```python
from build123d import *

# Parameters (mm, degrees)
PAD_DEPTH    = 6
PAD001_DEPTH = 5
SKETCH002_R  = 25
PAD002_DEPTH = 3
SKETCH003_R  = 20
PAD003_DEPTH = 12
FILLET_R     = 2


with BuildPart() as part:
    # Sketch → Pad (new body)
    with BuildSketch(Plane.XY):
        with BuildLine():
            Line((-1.45, 1.377498), (-1.45, -1.377498))
            ThreePointArc((-1.45, -1.377498), (0, -1.942662), (1.45, -1.377498))
            Line((1.45, 1.377498), (1.45, -1.377498))
            ThreePointArc((1.45, 1.377498), (0, 1.942662), (-1.45, 1.377498))
        make_face()
    extrude(amount=-PAD_DEPTH)

    # Sketch001 → Pad001 (join)
    with BuildSketch(Plane.XY):
        with BuildLine():
            Line((-8.25, 0), (0, 8.25))
            ThreePointArc((-8.25, 0), (5.833631, -5.833631), (0, 8.25))
        make_face()
    extrude(amount=PAD001_DEPTH)

    # Sketch002 → Pad002 (join)
    with BuildSketch(Plane.XY.offset(5)):
        Circle(SKETCH002_R)
    extrude(amount=PAD002_DEPTH)

    # Sketch003 → Pad003 (join)
    with BuildSketch(Plane.XY.offset(7)):
        Circle(SKETCH003_R)
    extrude(amount=PAD003_DEPTH)

    # Fillet
    fillet_edges = [part.edges().sort_by_distance(p)[0] for p in [
        (-20, 0, 19),
        (-20, 0, 8),
        (-25, 0, 8),
    ]]
    fillet(fillet_edges, radius=FILLET_R)


solid = part.part
```
The model under review builds one solid part; all positions refer to its coordinate system, in mm. A direction names the side the tool comes from. Give positions to 0.01 mm unless a question says otherwise; leave off trailing zeros. Write each loop counter-clockwise with the first axis right and the second up, starting at its lowest first coordinate (ties: lowest second). Pieces come first, ordered by that corner, then holes. Notation, with made-up numbers: M 4.5,24 L 9.5,24 A22 cw 9.5,54 Z; hole C -8.75,29.5 d10. An arc over 180 degrees is marked long. Answer in a Markdown table with one row per item.
Item 1: For P1, Ø4, axis at x = -6.5, z = 16, coming from the +Y side; P2, Ø3, axis at x = -3.5, y = -3.5, coming from the -Z side; P3, Ø6, axis at y = -14, z = 11.5, coming from the -X side; P4, Ø5, axis at x = 1.5, y = 1.5, coming from the -Z side, all flat-tipped, find the tip position at first contact; note any pin that passes through.
Check sheet entries:
| item | result |
|---|---|
| P1 | y = 19.49 |
| P2 | z = 0 |
| P3 | x = -16.7 |
| P4 | z = -6 |
Item 2: Add section A-A on z = -3.5. Give the boundary of the cut face in (x, y), plus the area to 3 significant figures.
Check sheet entries:
| item | result |
|---|---|
| outline | M -1.45,-1.38 A2.14 ccw 1.45,-1.38 L 1.45,1.38 A2.14 ccw -1.45,1.38 Z |
| area | 10.2 mm2 |
Item 3: For line 1 along Z through (x, y) = (-1.5, 3); line 2 along Z through (x, y) = (1.5, 14.5); line 3 along X through (y, z) = (0.5, -4.25), list the stretches that pass through material, from the lowest coordinate up.
Check sheet entries:
| item | result |
|---|---|
| line 1 | 0 to 19 |
| line 2 | 5 to 19 |
| line 3 | -1.45 to 1.45 |
Item 4: Add section B-B on z = 3. Give the boundary of the cut face in (x, y).
Check sheet entries:
| item | result |
|---|---|
| outline | M -8.25,0 A8.25 ccw long 0,8.25 Z |
Item 5: Tool access review of faces 1 (the face through (-4.18, 4.07, 2.46)), 2 (the face through (1.45, 0, -3)), 3 (the face through (-4.336, -19.524, 13.451)), 4 (the face through (-1.45, 0, -3)), 5 (the face through (0.022, 1.943, -2.958)): name each direction out of +Z, -Z, +X, -X, +Y, -Y from which nothing blocks a thin tool from reaching the whole face with its end or side.
Check sheet entries:
| item | result |
|---|---|
| face 1 | -Z, -X, +Y |
| face 2 | -Z, +X, +Y, -Y |
| face 3 | +Z |
| face 4 | -Z, -X, +Y, -Y |
| face 5 | -Z, +Y |
